Geometry check sheet. Reference: drawing and pictorial views, mm from the part's lowest x, y, z. A direction names the side the tool comes from. Coordinates: 2 decimals unless noted, no trailing zeros. Loops run counter-clockwise (first coordinate to the right, second up) from the corner with the lowest first, then second, coordinate; pieces in that order, holes last. Notation, with made-up numbers: M -11,68 L 48,68 A36 cw 48,104 Z; hole C -34,-14.5 d11. An arc over 180 degrees is marked long. Write each question's results on one line, items separated by ' | '. Start each with the question number.
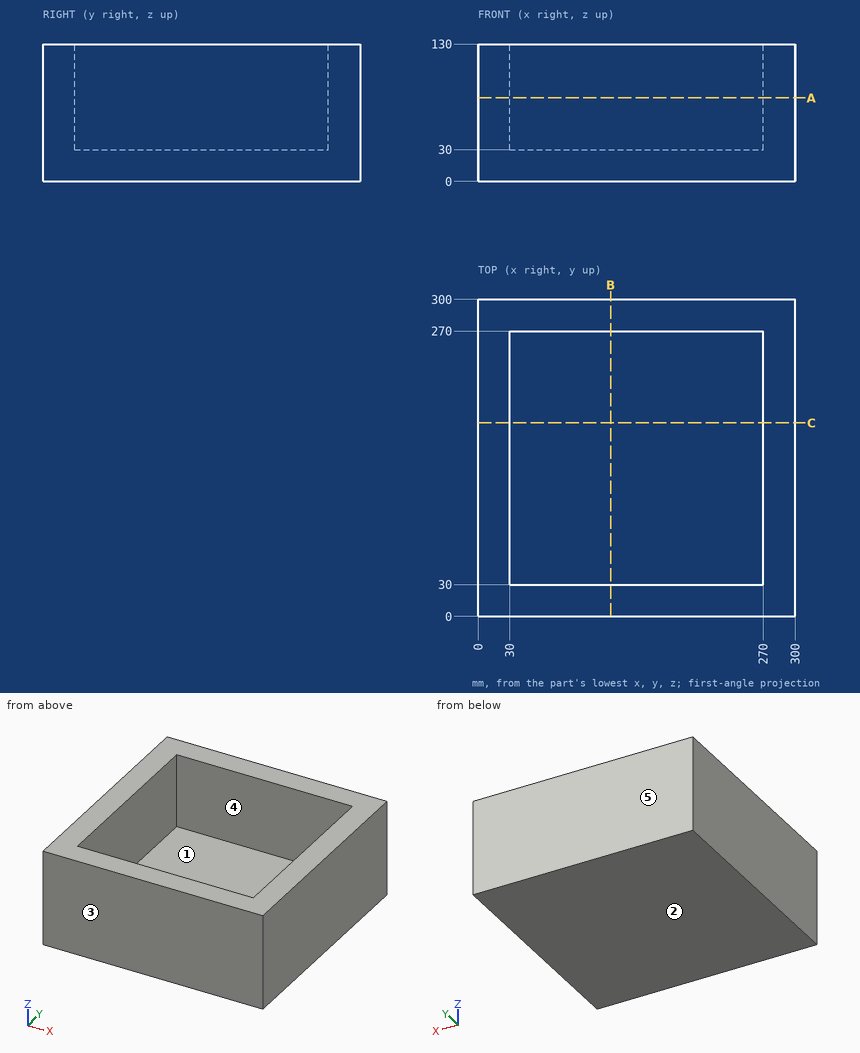
1) Gauge pin test, flat end, axial feed: P1, Ø12, axis at x = 237.5, y = 245.5, coming from the +Z side. Record the tip position at first contact, or that the pin passes through.
2) Thickness scan on probe 1 along X at (y, z) = (116, 96.5); probe 2 along Z at (x, y) = (260, 33.5). Record the ranges inside material, lowest first.
3) Release check for a two-part mould opening along Y. For the marked faces 1, 2 and 3 record: +Y half, -Y half, draft (parallel to the pull), parting line (faces both ways), or undercut.
4) Section check B-B (x = 125.5). Enter the section's corners in (y, z), then the cut area to 3 significant figures.
5) Set-up check for the marked faces 4 and 5: record each of +Z, -Z, +X, -X, +Y, -Y from which the full face is reachable in a straight line by a thin tool's end or side.
6) Section check A-A (z = 79). Enter the section's corners in (x, y), then the cut area to 3 significant figures.
Return value:
1) P1: stops at z = 30
2) probe 1: x = 0 to 30, 270 to 300 | probe 2: z = 0 to 30
3) face 1: undercut | face 2: draft | face 3: -Y half
4) outline: M 0,0 L 300,0 L 300,130 L 270,130 L 270,30 L 30,30 L 30,130 L 0,130 Z | area: 15,000 mm2
5) face 4: +Z | face 5: +Z, -Z, +X, -X, +Y
6) outline: M 0,0 L 300,0 L 300,300 L 0,300 Z; hole M 30,30 L 270,30 L 270,270 L 30,270 Z | area: 32,400 mm2
